The model under review builds one solid part; all positions refer to its coordinate system, in mm. A direction names the side the tool comes from. Round coordinates to 2 decimals unless told otherwise and drop trailing zeros. Order: outer loops, then holes, each group sorted by start corner. A loop starts at its lowest first (then second) coordinate and runs counter-clockwise, first axis right, second up. Notation, with made-up numbers: M -3,77 L 6,77 A30 ccw 6,115 Z; hole C 28,-33.75 d2. An arc over 180 degrees is marked long. Answer as a JSON object with one key per item and string values. Group by question number.
1. Add section B-B on z = 70. State the section outline as (x, y) points, and give its area (3 significant figures).
2. To check wall thickness, follow probe 1 along Z at (x, y) = (2.4, 0); probe 2 along Z at (x, y) = (2.3, -3); probe 3 along Y at (x, z) = (1.15, -52). State the ranges of each line that lie inside material, in increasing order. Write a range as [from, to].
3. Mouldability with a two-part tool opening along Y and no side actions: class faces 1 (the face through (2.54, 29.6, -29.14)), 2 (the face through (2, 21, -30)), 3 (the face through (2.535, 12.973, 24.859)) as released by +Y, released by -Y, zero draft, split by the parting line, or undercut.
4. Add section C-C on x = 4.25. State the section outline as (y, z) points.
5. Machinability: for faces 4 (the face through (2.535, -3.358, 25.727)), 5 (the face through (2, 23, 30)), which of the approach directions +Z, -Z, +X, -X, +Y, -Y give a long, thin tool a straight path to every point of the face, cutting with its end or side? Answer none if there is none.
6. Add section A-A on y = 7.5. State the section outline as (x, z) points, and give its area (3 significant figures).
7. Clearance check with flat-ended pins moving along their axes: P1, Ø5, axis at y = -3, z = 23, coming from the +X side; P2, Ø2.5, axis at x = 3.5, y = 18.5, coming from the -Z side; P3, Ø1.5, axis at x = 2.5, y = 23.5, coming from the +Z side. State where each tip first meets the part, or that it passes through.
8. Add section D-D on z = -23. State the section outline as (x, y) points.
```python
from build123d import *

# Parameters (mm, degrees)
F1_DEPTH = 5
F2_R     = 3
F3_R     = 3.5
F4_DEPTH = 5
F6_R     = 12.5
F6_R_2   = 2.75
F7_DEPTH = 5


# Not quite as in the source:
# - two fillets or chamfers of one size are made in one step


with BuildPart() as f1:
    # F0 (on Right) → F1 (new body)
    with BuildSketch(Plane.YZ):
        Polygon((15, 30), (15, 85), (-15, 85), (-15, -85), (15, -85), (15, -30), (30.5, -30), (30.5, 30), align=None)
    extrude(amount=F1_DEPTH)

    # F2
    f2_edges = [f1.edges().sort_by_distance(p)[0] for p in [
        (2.5, -15, 85),
        (2.5, 15, 85),
        (2.5, -15, -85),
        (2.5, 15, 30),
        (2.5, 15, -85),
        (2.5, 30.5, -30),
        (2.5, 30.5, 30),
    ]]
    fillet(f2_edges, radius=F2_R)

    # F3 (on face) → F4 (cut)
    with BuildSketch(Plane.YZ.offset(5)):
        with Locations((0, 70)):
            Circle(F3_R)
        with Locations((0, -70)):
            Circle(F3_R)
    extrude(amount=-F4_DEPTH, mode=Mode.SUBTRACT)

    # F6 (on face) → F7 (cut)
    with BuildSketch(Plane.YZ.offset(5)):
        with Locations((15, 0)):
            Circle(F6_R)
        with Locations((15, 23)):
            Circle(F6_R_2)
        with Locations((15, -23)):
            Circle(F6_R_2)
        with Locations((-3, -23)):
            Circle(F6_R_2)
        with Locations((-3, 23)):
            Circle(F6_R_2)
    extrude(amount=-F7_DEPTH, mode=Mode.SUBTRACT)


solid = f1.part
```
Recorded:
{
 "1": {"outline": "M 0,-15 L 5,-15 L 5,-3.5 L 0,-3.5 Z; M 0,3.5 L 5,3.5 L 5,15 L 0,15 Z", "area": "115 mm²"},
 "2": {"probe 1": "z = [-85, -73.5], [-66.5, 66.5], [73.5, 85]", "probe 2": "z = [-85, -71.8], [-68.2, -25.75], [-20.25, 20.25], [25.75, 68.2], [71.8, 85]", "probe 3": "y = [-15, 15]"},
 "3": {"face 1": "released by +Y", "face 2": "zero draft", "face 3": "undercut"},
 "4": {"outline": "M -15,-82 A3 ccw -12,-85 L 12,-85 A3 ccw 15,-82 L 15,-30 L 27.5,-30 A3 ccw 30.5,-27 L 30.5,27 A3 ccw 27.5,30 L 18,30 A3 cw 15,33 L 15,82 A3 ccw 12,85 L -12,85 A3 ccw -15,82 Z; hole C -3,-23 d5.5; hole C -3,23 d5.5; hole C 0,-70 d7; hole C 0,70 d7; hole C 15,0 d25; hole C 15,-23 d5.5; hole C 15,23 d5.5"},
 "5": {"face 4": "+X, -X", "face 5": "+Z, +X, -X, +Y"},
 "6": {"outline": "M 0,-85 L 5,-85 L 5,-10 L 0,-10 Z; M 0,10 L 5,10 L 5,85 L 0,85 Z", "area": "750 mm²"},
 "7": {"P1": "passes through", "P2": "stops at z = -30", "P3": "stops at z = 30"},
 "8": {"outline": "M 0,-15 L 5,-15 L 5,-5.75 L 0,-5.75 Z; M 0,-0.25 L 5,-0.25 L 5,12.25 L 0,12.25 Z; M 0,17.75 L 5,17.75 L 5,30.5 L 0,30.5 Z"}
}
